Work out the finished part from the listing and answer in its coordinate system (mm). A direction names the side the tool comes from. Give positions to 0.01 mm unless a question says otherwise; leave off trailing zeros. Loops run counter-clockwise (first coordinate to the right, second up) from the corner with the lowest first, then second, coordinate; pieces in that order, holes last. Notation, with made-up numbers: (-1.5, 25) - (40.5, 25) arc R17 ccw to (40.5, 46) - close; hole circle Ø3 at (45.5, -15). An arc over 180 degrees is marked (long way). One line per question, with ' | ' between items. Start each with the question number.
1. Find the intervals of material crossed by line 1 (Y direction, x = 0.75, z = 6.75); line 2 (Y direction, x = 7, z = 3); line 3 (X direction, y = -14.5, z = -0.25), in increasing order.
2. For a pull along Y with two mould halves and no side action, classify faces 1 (the face through (0, -19, -9)), 2 (the face through (2, -12.25, -6)), 3 (the face through (7, -16.75, 3)) as released by +Y, released by -Y, zero draft, split by the parting line, or undercut.
3. Each of these flat-tipped pins is pushed along its axis until it touches: pin 1 (6 mm diameter, centred on x = 2, y = 6, fed in from -Z); pin 2 (1.5 mm diameter, centred on x = 1.5, y = 1, fed in from -Z); pin 3 (2 mm diameter, centred on x = 4, z = -4.5, fed in from +Y). Where does it stop, or does it pass through?
4. Which of the six approach directions +Z, -Z, +X, -X, +Y, -Y give full straight-line access (tool end or side, diameter ignored) to faces 4 (the face through (-5.604, -14.236, -1.765)), 5 (the face through (0, 10.55, 0)), 6 (the face through (5.08, -1.29, 3.89))?
5. Section A-A (y = 4.5) is taken. Determine the outline of the cut face in (x, z), plus the area to 3 significant figures.
from build123d import *

# Parameters (mm, degrees)
ENL_V_MAT_EXTRU_1_DEPTH = 35.71728676
CHANFREIN1_SIZE         = 0.65


with BuildPart() as part:
    # Esquisse1 → Révolution1 (revolve)
    with BuildSketch(Plane.XY):
        Polygon((0, -21.75), (-9, -21.75), (-9, -16.75), (-7.05, -16.75), (-7.05, -15.25), (-5.875, -15.25), (-5.875, -13.25), (-7.05, -13.25), (-7.05, -12.25), (-5.875, -12.25), (-5.875, -10.25), (-7.05, -10.25), (-7.05, -7.7), (-6.4, -7.7), (-6.4, -6.05), (-7, -6.05), (-7, -1.95), (-6.4, -1.95), (-6.4, 0), (-2.5, 0), (-2.5, 10.55), (0, 10.55), (0, 0), align=None)
    revolve(axis=Axis((0, 0, 0), (0, -1, 0)))

    # Esquisse2 → Enlèv. mat.-Extru.1 (cut, through all)
    with BuildSketch(Plane.XZ.offset(21.75)):
        with BuildLine():
            Line((8, 4.123105626), (8, -4.123105626))
            ThreePointArc((8, -4.123105626), (9, 0), (8, 4.123105626))
        make_face()
        with BuildLine():
            Line((-8, 4.123105626), (-8, -4.123105626))
            ThreePointArc((-8, -4.123105626), (-9, 0), (-8, 4.123105626))
        make_face()
    extrude(amount=-ENL_V_MAT_EXTRU_1_DEPTH, mode=Mode.SUBTRACT)

    # Chanfrein1
    chanfrein1_edges = [part.edges().sort_by_distance(p)[0] for p in [
        (2.5, 10.55, 0),
        (6.4, 0, 0),
        (7.05, -7.7, 0),
    ]]
    chamfer(chanfrein1_edges, length=CHANFREIN1_SIZE - 0.0001)  # a hair under: the kernel refuses the full size


solid = part.part
Conclusion:
1) line 1: -21.75 to -15.25, -13.25 to -12.25, -10.25 to -8.09, -6.05 to -1.95 | line 2: -21.75 to -16.75 | line 3: -5.87 to 5.87
2) face 1: zero draft | face 2: undercut | face 3: released by +Y
3) pin 1: z = -2.5 | pin 2: z = -2.38 | pin 3: y = 0
4) face 4: none | face 5: +Z, -Z, +X, -X, +Y | face 6: +Y
5) outline: circle Ø5 at (0, 0) | area: 19.6 mm²
